Autodesk Inventor part; units mm, degrees
ref_plane "YZ Plane" through (0, 0, 0) normal (1, 0, 0) x (0, 1, 0)
ref_plane "XZ Plane" through (0, 0, 0) normal (0, 1, 0) x (-1, 0, 0)
ref_plane "XY Plane" through (0, 0, 0) normal (0, 0, 1) x (1, 0, 0)
sketch "Sketch1" plane through (0, 0, 0) normal (0, 1, 0) x (-1, 0, 0)
  circle A0 centre (29.9915, -10) radius 2.75
  circle A1 centre (9.9915, -10) radius 2.75
  line L0 (0, 0) -> (0, -6.5)
  line L1 (-0.0085, -20) -> (-0.0085, -13.5)
  line L2 (0, -6.5) -> (0.5, -6.5)
  line L3 (0.5, -6.5) -> (0.5, -7)
  line L4 (0.5, -7) -> (1, -7)
  line L5 (-0.0085, -13.5) -> (0.4915, -13.5)
  line L6 (0.4915, -13.5) -> (0.4915, -13)
  line L7 (0.4915, -13) -> (0.9915, -13)
  line L8 (1, -4.05) -> (3, -4.05)
  line L9 (0.9915, -15.95) -> (2.9915, -15.95)
  line L10 (5.5, -6.5) -> (5.5, -13.5)
  line L11 (5.5, -13.5) -> (2.9915, -15.95)
  line L12 (5.5, -6.5) -> (3, -4.05)
  line L13 (1, -4.05) -> (1, -7)
  line L14 (0.9915, -13) -> (0.9915, -15.95)
  line L15 (-0.0085, -20) -> (6.4915, -20)
  line L16 (6.4915, -20) -> (6.4915, -19.5)
  line L17 (6.4915, -19.5) -> (6.9915, -19.5)
  line L18 (6.9915, -19.5) -> (6.9915, -19)
  line L19 (6.9915, -19) -> (4.0415, -19)
  line L20 (4.0415, -19) -> (4.0415, -17)
  line L21 (13.4915, -20) -> (13.4915, -19.5)
  line L22 (13.4915, -19.5) -> (12.9915, -19.5)
  line L23 (12.9915, -19.5) -> (12.9915, -19)
  line L24 (12.9915, -19) -> (15.9415, -19)
  line L25 (15.9415, -19) -> (15.9415, -17)
  line L26 (15.9415, -17) -> (13.4915, -14.5)
  line L27 (6.4915, -14.5) -> (13.4915, -14.5)
  line L28 (4.0415, -17) -> (6.4915, -14.5)
  line L29 (39.9915, 0) -> (39.9915, -6.5)
  line L30 (39.9915, -6.5) -> (39.4915, -6.5)
  line L31 (39.4915, -6.5) -> (39.4915, -7)
  line L32 (39.4915, -7) -> (38.9915, -7)
  line L33 (38.9915, -7) -> (38.9915, -4.05)
  line L34 (38.9915, -4.05) -> (36.9915, -4.05)
  line L35 (39.9915, -20) -> (39.9915, -13.5)
  line L36 (39.9915, -13.5) -> (39.4915, -13.5)
  line L37 (39.4915, -13.5) -> (39.4915, -13)
  line L38 (39.4915, -13) -> (38.9915, -13)
  line L39 (38.9915, -13) -> (38.9915, -15.95)
  line L40 (38.9915, -15.95) -> (36.9915, -15.95)
  line L41 (34.4915, -6.601) -> (34.4915, -13.5)
  line L42 (34.4915, -13.5) -> (36.9915, -15.95)
  line L43 (34.4915, -6.601) -> (36.9915, -4.05)
  line L44 (39.9915, -20) -> (33.4915, -20)
  line L45 (33.4915, -20) -> (33.4915, -19.5)
  line L46 (33.4915, -19.5) -> (32.9915, -19.5)
  line L47 (32.9915, -19.5) -> (32.9915, -19)
  line L48 (32.9915, -19) -> (35.9415, -19)
  line L49 (35.9415, -19) -> (35.9415, -17)
  line L50 (26.4915, -20) -> (26.4915, -19.5)
  line L51 (26.4915, -19.5) -> (26.9915, -19.5)
  line L52 (26.9915, -19.5) -> (26.9915, -19)
  line L53 (26.9915, -19) -> (24.0415, -19)
  line L54 (24.0415, -19) -> (24.0415, -17)
  line L55 (33.4915, -14.5) -> (26.4915, -14.5)
  line L56 (24.0415, -17) -> (26.4915, -14.5)
  line L57 (33.4915, -14.5) -> (35.9415, -17)
  line L58 (26.4915, -20) -> (13.4915, -20)
  line L59 (39.9915, 0) -> (33.4915, 0)
  line L60 (33.4915, 0) -> (33.4915, -0.5)
  line L61 (33.4915, -0.5) -> (32.9915, -0.5)
  line L62 (32.9915, -0.5) -> (32.9915, -1)
  line L63 (32.9915, -1) -> (35.9415, -1)
  line L64 (35.9415, -1) -> (35.9415, -3)
  line L65 (26.4915, 0) -> (26.4915, -0.5)
  line L66 (26.4915, -0.5) -> (26.9915, -0.5)
  line L67 (26.9915, -0.5) -> (26.9915, -1)
  line L68 (26.9915, -1) -> (24.0415, -1)
  line L69 (24.0415, -1) -> (24.0415, -3)
  line L70 (33.4915, -5.5) -> (26.4915, -5.5)
  line L71 (24.0415, -3) -> (26.4915, -5.5)
  line L72 (35.9415, -3) -> (33.4915, -5.5)
  line L73 (0, 0) -> (6.5, 0)
  line L74 (6.5, 0) -> (6.5, -0.5)
  line L75 (6.5, -0.5) -> (7, -0.5)
  line L76 (7, -0.5) -> (7, -1)
  line L77 (7, -1) -> (4.05, -1)
  line L78 (4.05, -1) -> (4.05, -3)
  line L79 (13.5, 0) -> (13.5, -0.5)
  line L80 (13.5, -0.5) -> (13, -0.5)
  line L81 (13, -0.5) -> (13, -1)
  line L82 (13, -1) -> (15.95, -1)
  line L83 (15.95, -1) -> (15.95, -3)
  line L84 (13.5, -5.5) -> (6.5, -5.5)
  line L85 (6.5, -5.5) -> (4.05, -3)
  line L86 (15.95, -3) -> (13.5, -5.5)
  line L87 (13.5, 0) -> (26.4915, 0)
  dimension "d0" = 40
  dimension "d1" = 20
  dimension "d2" = 5.5
  dimension "d3" = 5.5
  dimension "d4" = 20
  dimension "d11" = 6.5
  dimension "d12" = 6.5
  dimension "d13" = 0.5
  dimension "d14" = 0.5
  dimension "d15" = 0.5
  dimension "d16" = 0.5
  dimension "d17" = 0.5
  dimension "d18" = 0.5
  dimension "d19" = 5.5
  dimension "d20" = 11.9
  dimension "d21" = 6.5
  dimension "d22" = 0.5
  dimension "d23" = 0.5
  dimension "d24" = 0.5
  dimension "d25" = 0.5
  dimension "d26" = 0.5
  dimension "d27" = 0.5
  dimension "d28" = 7
  dimension "d29" = 11.9
  dimension "d31" = 4.05
  dimension "d32" = 2.95
  dimension "d34" = 2
  dimension "d35" = 2
  dimension "d36" = 2
  dimension "d37" = 2
  dimension "d39" = 7
  dimension "d40" = 6.5
  dimension "d41" = 0.5
  dimension "d42" = 0.5
  dimension "d43" = 0.5
  dimension "d44" = 2.95
  dimension "d45" = 2
  dimension "d46" = 6.5
  dimension "d47" = 0.5
  dimension "d48" = 0.5
  dimension "d49" = 0.5
  dimension "d50" = 2.95
  dimension "d51" = 2
  dimension "d52" = 5.5
  dimension "d53" = 6.5
  dimension "d54" = 0.5
  dimension "d55" = 0.5
  dimension "d56" = 0.5
  dimension "d57" = 2.95
  dimension "d58" = 2
  dimension "d59" = 0.5
  dimension "d60" = 0.5
  dimension "d61" = 0.5
  dimension "d62" = 2.95
  dimension "d63" = 2
  dimension "d64" = 7
  dimension "d66" = 6.5
  dimension "d67" = 0.5
  dimension "d68" = 0.5
  dimension "d69" = 0.5
  dimension "d70" = 2.95
  dimension "d71" = 2
  dimension "d72" = 0.5
  dimension "d73" = 0.5
extrude "Extrusion1" add sketch "Sketch1" along normal blind 508
properties part number "Tslot_2040extrusion_20inch"
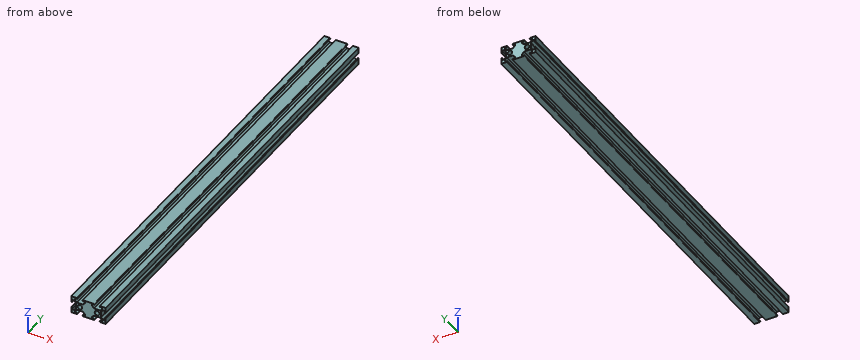
Geometry: final body of the model. Coordinates: model frame, mm. Give positions to 0.01 mm unless a question says otherwise; leave off trailing zeros. Put each result on its own line as item: value.
1. Ray query, line 1 along X through (y, z) = (177, -9.5); line 2 along X through (y, z) = (208.5, -18); line 3 along Z through (x, y) = (-10, 346). Return the intervals inside material, ascending. Write a range as [from, to].
Taken from the geometry:
line 1: x = [-34.49, -32.7], [-27.29, -12.7], [-7.29, -5.5]
line 2: x = [-39.99, -35.94], [-24.04, -15.94], [-4.04, 0.01]
line 3: z = [-14.5, -12.75], [-7.25, -5.5]
2. Pin query (flat end, axial travel): P1, Ø3, axis at y = 371, z = -11, coming from the -X side; P2, Ø1.6, axis at y = 287.5, z = -2, coming from the +X side; P3, Ø3.5, axis at x = -10.5, y = 270, coming from the +Z side. Return the tip coordinate at first contact, or that it passes through.
Taken from the geometry:
P1: stops at x = -34.49
P2: stops at x = 0
P3: stops at z = -5.5
3. Cut plane A-A (y = 155). Count the separate pieces of the cut face and the enclosed holes in it, plus the area to 3 significant figures.
Taken from the geometry:
separate pieces: 1
enclosed holes: 2
area: 429 mm2
